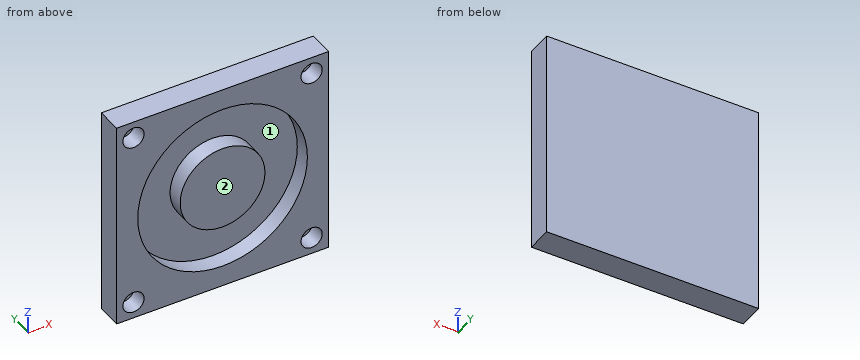
from build123d import *

# Parameters (mm, degrees)
SKETCH1_W           = 25
SKETCH1_H           = 25
BOSS_EXTRUDE1_DEPTH = 3
SKETCH2_R           = 10
SKETCH2_R_2         = 5
CUT_EXTRUDE1_DEPTH  = 2
SKETCH3_R           = 1.25
CUT_EXTRUDE2_DEPTH  = 2


with BuildPart() as part:
    # Sketch1 → Boss-Extrude1 (new body)
    with BuildSketch(Plane(origin=(0, 0, 0), x_dir=(1, 0, 0), z_dir=(0, 1, 0))):
        Rectangle(SKETCH1_W, SKETCH1_H)
    extrude(amount=BOSS_EXTRUDE1_DEPTH)

    # Sketch2 → Cut-Extrude1 (cut)
    with BuildSketch(Plane.XZ):
        Circle(SKETCH2_R)
        Circle(SKETCH2_R_2, mode=Mode.SUBTRACT)
    extrude(amount=-CUT_EXTRUDE1_DEPTH, mode=Mode.SUBTRACT)

    # Sketch3 → Cut-Extrude2 (cut)
    with BuildSketch(Plane.XZ):
        with Locations((-10.5, 10.5)):
            Circle(SKETCH3_R)
        with Locations((10.5, 10.5)):
            Circle(SKETCH3_R)
        with Locations((10.5, -10.5)):
            Circle(SKETCH3_R)
        with Locations((-10.5, -10.5)):
            Circle(SKETCH3_R)
    extrude(amount=-CUT_EXTRUDE2_DEPTH, mode=Mode.SUBTRACT)


solid = part.part
Verification items for the finished model (mm, model axes). Face numbers are marked on the shaded views. Coordinates: 2 decimals unless noted, no trailing zeros. Order: outer loops, then holes, each group sorted by start corner. A loop starts at its lowest first (then second) coordinate and runs counter-clockwise, first axis right, second up. Notation, with made-up numbers: M 8.5,30 L 38.5,30 A12 ccw 38.5,49 Z; hole C 3,80 d3. An arc over 180 degrees is marked long. Write each question's results on one line, items separated by ' | '.
1) Section check B-B on z = -10.5. Record the cut outline in (x, y).
Solved:
outline: M -12.5,0 L -11.75,0 L -11.75,2 L -9.25,2 L -9.25,0 L 9.25,0 L 9.25,2 L 11.75,2 L 11.75,0 L 12.5,0 L 12.5,3 L -12.5,3 Z
2) Scan lines: line 1 along Z through (x, y) = (-10.5, 0.8); line 2 along Z through (x, y) = (-1.75, 0.4); line 3 along X through (y, z) = (1.3, -1.25). Record each from-to range of solid material in increasing order. Write a range as [from, to].
Solved:
line 1: z = [-12.5, -11.75], [-9.25, 9.25], [11.75, 12.5] | line 2: z = [-12.5, -9.85], [-4.68, 4.68], [9.85, 12.5] | line 3: x = [-12.5, -9.92], [-4.84, 4.84], [9.92, 12.5]
3) Release check for a two-part mould opening along X. For the marked faces 1 and 2 record: pulls with the +X half, pulls with the -X half, needs draft (parallel to the pull), parting line crosses it, or undercut.
Solved:
face 1: undercut | face 2: needs draft
4) Section check A-A on y = 1.3. Record the cut outline in (x, z).
Solved:
outline: M -12.5,-12.5 L 12.5,-12.5 L 12.5,12.5 L -12.5,12.5 Z; C 0,0 d10; hole C -10.5,-10.5 d2.5; hole C -10.5,10.5 d2.5; hole C 0,0 d20; hole C 10.5,-10.5 d2.5; hole C 10.5,10.5 d2.5
5) Gauge pin test, flat end, axial feed: pin 1 Ø1.2 at (x, z) = (-10.5, -10.5) entering from -Y. Record the tip position at first contact, or that the pin passes through.
Solved:
pin 1: stops at y = 2
6) Section check C-C on x = 0. Record the cut outline in (y, z), plus the area to 3 significant figures.
Solved:
outline: M 0,-12.5 L 3,-12.5 L 3,12.5 L 0,12.5 L 0,10 L 2,10 L 2,5 L 0,5 L 0,-5 L 2,-5 L 2,-10 L 0,-10 Z | area: 55.0 mm²
7) Section check D-D on x = 8.25. Record the cut outline in (y, z), plus the area to 3 significant figures.
Solved:
outline: M 0,-12.5 L 3,-12.5 L 3,12.5 L 0,12.5 L 0,5.65 L 2,5.65 L 2,-5.65 L 0,-5.65 Z | area: 52.4 mm²
